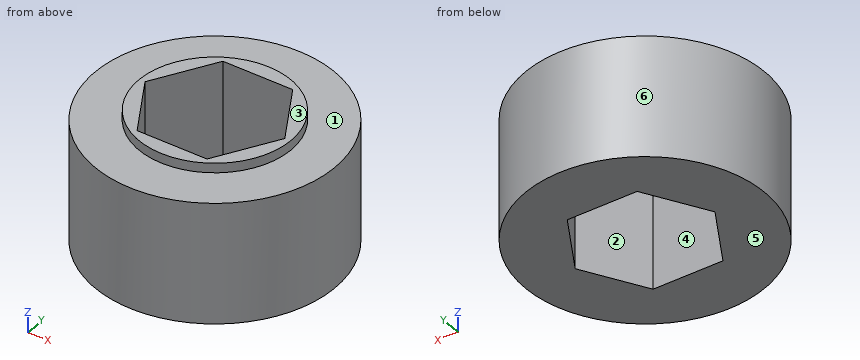
```python
from build123d import *

# Parameters (mm, degrees)
SKETCH1_R           = 12.5
BOSS_EXTRUDE1_DEPTH = 6.8
SKETCH2_R           = 12.5
SKETCH2_R_2         = 7.9375
CUT_EXTRUDE1_DEPTH  = 1


with BuildPart() as part:
    # Sketch1 → Boss-Extrude1 (new, symmetric)
    with BuildSketch(Plane.XY):
        Circle(SKETCH1_R)
        Polygon((7.332348419, 0), (3.666174209, 6.35), (-3.666174209, 6.35), (-7.332348419, 0), (-3.666174209, -6.35), (3.666174209, -6.35), align=None, mode=Mode.SUBTRACT)
    extrude(amount=BOSS_EXTRUDE1_DEPTH, both=True)

    # Sketch2 → Cut-Extrude1 (cut)
    with BuildSketch(Plane.XY.offset(6.8)):
        Circle(SKETCH2_R)
        Circle(SKETCH2_R_2, mode=Mode.SUBTRACT)
    extrude(amount=-CUT_EXTRUDE1_DEPTH, mode=Mode.SUBTRACT)


solid = part.part
```
CAD build for the part. Positions are in the model's coordinates, mm. Face numbers are marked on the shaded views. A direction names the side the tool comes from. Round coordinates to 2 decimals unless told otherwise and drop trailing zeros. Write each loop counter-clockwise with the first axis right and the second up, starting at its lowest first coordinate (ties: lowest second). Pieces come first, ordered by that corner, then holes. Notation, with made-up numbers: (25, 76.25) - (65, 76.25) arc R15 cw to (65, 91.25) - close; hole circle Ø3 at (22.25, 36). An arc over 180 degrees is marked (long way). Return JSON: item names as keys, results as strings. Group by question number.
Item 1: Probe probe 1 along Z at (x, y) = (-9.75, 1); probe 2 along Y at (x, z) = (7.25, -4.5); probe 3 along Y at (x, z) = (-5.5, 3). List the from-to ranges inside material, lowest first.
Item 2: Band-saw the part on D-D on x = 9.5. List the corners of the cut face in (y, z), plus the area to 3 significant figures.
Item 3: Band-saw the part on A-A on x = 0. List the corners of the cut face in (y, z), plus the area to 3 significant figures.
Item 4: Mould opens along X. For the marked faces 4, 5 and 6 say: +X half, -X half, draft (parallel to the pull), parting line (faces both ways), or undercut.
Item 5: Band-saw the part on C-C on y = 5.75. List the corners of the cut face in (x, z), plus the area to 3 significant figures.
Item 6: 3-axis set-ups, long thin cutter, end or side, ignore diameter. For the marked faces 1, 2 and 3: which of +Z, -Z, +X, -X, +Y, -Y reach the whole face in a straight line?
Item 7: Flat gauge pins, fed straight in: pin 1 Ø1.5 at (y, z) = (10, -3) entering from -X; pin 2 Ø8 at (y, z) = (-9, 2.5) entering from +X; pin 3 Ø2 at (x, z) = (-2.5, 1.5) entering from +Y; pin 4 Ø8 at (x, z) = (1.5, -2) entering from -Y. Where does each tip first touch, or does it go through?
Item 8: Band-saw the part on B-B on z = -0.5. List the corners of the cut face in (x, y), plus the area to 3 significant figures.
Resolved:
{
 "1": {"probe 1": "z = -6.8 to 5.8", "probe 2": "y = -10.18 to -0.14, 0.14 to 10.18", "probe 3": "y = -11.22 to -3.17, 3.17 to 11.22"},
 "2": {"outline": "(-8.12, -6.8) - (8.12, -6.8) - (8.12, 5.8) - (-8.12, 5.8) - close", "area": "205 mm²"},
 "3": {"outline": "(-12.5, -6.8) - (-6.35, -6.8) - (-6.35, 6.8) - (-7.94, 6.8) - (-7.94, 5.8) - (-12.5, 5.8) - close; (6.35, -6.8) - (12.5, -6.8) - (12.5, 5.8) - (7.94, 5.8) - (7.94, 6.8) - (6.35, 6.8) - close", "area": "158 mm²"},
 "4": {"face 4": "undercut", "face 5": "draft", "face 6": "parting line"},
 "5": {"outline": "(-11.1, -6.8) - (-4.01, -6.8) - (-4.01, 6.8) - (-5.47, 6.8) - (-5.47, 5.8) - (-11.1, 5.8) - close; (4.01, -6.8) - (11.1, -6.8) - (11.1, 5.8) - (5.47, 5.8) - (5.47, 6.8) - (4.01, 6.8) - close", "area": "181 mm²"},
 "6": {"face 1": "+Z", "face 2": "+Z, -Z", "face 3": "+Z, +X, -X, +Y, -Y"},
 "7": {"pin 1": "stops at x = -8.41", "pin 2": "stops at x = 11.46", "pin 3": "stops at y = 12.41", "pin 4": "stops at y = -12.5"},
 "8": {"outline": "circle Ø25 at (0, 0); hole (-7.33, 0) - (-3.67, -6.35) - (3.67, -6.35) - (7.33, 0) - (3.67, 6.35) - (-3.67, 6.35) - close", "area": "351 mm²"}
}
